from build123d import *

# Parameters (mm, degrees)
F0_R     = 11.2522
F1_DEPTH = 8.636


with BuildPart() as f1:
    # F0 (on Top) → F1 (new body)
    with BuildSketch(Plane.XY):
        with BuildLine():
            ThreePointArc((10.0592163849, -12.5427541219), (14.4955615296, -6.9560916599), (16.0782, 0))
            ThreePointArc((16.0782, 0), (15.9356487874, 2.1362614454), (15.5105229014, 4.2346422002))
            ThreePointArc((15.5105229014, 4.2346422002), (15.2912768803, 4.968437039), (15.0373368529, 5.6909591117))
            ThreePointArc((15.0373368529, 5.6909591117), (9.4505288434, 13.007537039), (0.7656311095, 16.0599602815))
            ThreePointArc((0.7656311095, 16.0599602815), (0, 16.0782), (-0.7656311095, 16.0599602815))
            ThreePointArc((-0.7656311095, 16.0599602815), (-9.4505288434, 13.007537039), (-15.0373368529, 5.6909591117))
            ThreePointArc((-15.0373368529, 5.6909591117), (-15.2912768803, 4.968437039), (-15.5105229014, 4.2346422002))
            ThreePointArc((-15.5105229014, 4.2346422002), (-15.2912768803, -4.968437039), (-10.0592163849, -12.5427541219))
            ThreePointArc((-10.0592163849, -12.5427541219), (-9.4505288434, -13.007537039), (-8.8203992269, -13.4428074716))
            ThreePointArc((-8.8203992269, -13.4428074716), (0, -16.0782), (8.8203992269, -13.4428074716))
            ThreePointArc((8.8203992269, -13.4428074716), (9.4505288434, -13.007537039), (10.0592163849, -12.5427541219))
        make_face()
        Circle(F0_R, mode=Mode.SUBTRACT)
        with BuildLine():
            ThreePointArc((0.7656311095, 16.0599602815), (9.4505288434, 13.007537039), (15.0373368529, 5.6909591117))
            ThreePointArc((15.0373368529, 5.6909591117), (15.1741938942, 5.3328401038), (15.3133632508, 4.9756133358))
            ThreePointArc((15.3133632508, 4.9756133358), (13.983030327, 11.6776288921), (13.4324519852, 18.4881840601))
            ThreePointArc((13.4324519852, 18.4881840601), (6.7850910488, 16.9072378917), (0, 16.1014229843))
            ThreePointArc((0, 16.1014229843), (0.3827485418, 16.079454203), (0.7656311095, 16.0599602815))
        make_face()
        with BuildLine():
            ThreePointArc((15.5105229014, 4.2346422002), (15.9356487874, 2.1362614454), (16.0782, 0))
            ThreePointArc((16.0782, 0), (14.4955615296, -6.9560916599), (10.0592163849, -12.5427541219))
            ThreePointArc((10.0592163849, -12.5427541219), (9.7609161203, -12.7835777623), (9.4641789711, -13.0263248279))
            ThreePointArc((9.4641789711, -13.0263248279), (15.4270790567, -9.6900663284), (21.7341638644, -7.0618579207))
            ThreePointArc((21.7341638644, -7.0618579207), (18.176447212, -1.2283812192), (15.3133632508, 4.9756133358))
            ThreePointArc((15.3133632508, 4.9756133358), (15.4107455022, 4.6048091142), (15.5105229014, 4.2346422002))
        make_face()
        with BuildLine():
            ThreePointArc((13.4324519852, 18.4881840601), (13.983030327, 11.6776288921), (15.3133632508, 4.9756133358))
            ThreePointArc((15.3133632508, 4.9756133358), (18.176447212, -1.2283812192), (21.7341638644, -7.0618579207))
            ThreePointArc((21.7341638644, -7.0618579207), (30.0130318433, -4.8169203604), (38.5291644649, -3.789844495))
            ThreePointArc((38.5291644649, -3.789844495), (22.4722564751, 7.3016787476), (28.9431341285, 25.7129232581))
            ThreePointArc((28.9431341285, 25.7129232581), (21.4497380646, 21.5381879262), (13.4324519852, 18.4881840601))
        make_face()
        with BuildLine():
            ThreePointArc((53.8417333554, 12.2701157865), (45.4020008846, 26.4179894446), (28.9431341285, 25.7129232581))
            ThreePointArc((28.9431341285, 25.7129232581), (22.4722564751, 7.3016787476), (38.5291644649, -3.789844495))
            ThreePointArc((38.5291644649, -3.789844495), (49.4000810682, 1.1751046298), (53.8417333554, 12.2701157865))
        make_face()
        with Locations((37.7635333554, 12.2701157865)):
            Circle(F0_R, mode=Mode.SUBTRACT)
        with BuildLine():
            ThreePointArc((21.7341638644, -7.0618579207), (15.4270790567, -9.6900663284), (9.4641789711, -13.0263248279))
            ThreePointArc((9.4641789711, -13.0263248279), (4.4485711229, -17.6664192363), (0, -22.8526522788))
            ThreePointArc((0, -22.8526522788), (4.693373395, -30.0325997603), (8.301810296, -37.8145392867))
            ThreePointArc((8.301810296, -37.8145392867), (13.8886183055, -19.1160431361), (33.3983635338, -19.5808260531))
            ThreePointArc((33.3983635338, -19.5808260531), (27.1123675633, -13.7442470619), (21.7341638644, -7.0618579207))
        make_face()
        with BuildLine():
            ThreePointArc((9.4641789711, -13.0263248279), (9.1416159705, -13.2335256587), (8.8203992269, -13.4428074716))
            ThreePointArc((8.8203992269, -13.4428074716), (0, -16.0782), (-8.8203992269, -13.4428074716))
            ThreePointArc((-8.8203992269, -13.4428074716), (-9.1416159705, -13.2335256587), (-9.4641789711, -13.0263248279))
            ThreePointArc((-9.4641789711, -13.0263248279), (-4.4485711229, -17.6664192363), (0, -22.8526522788))
            ThreePointArc((0, -22.8526522788), (4.4485711229, -17.6664192363), (9.4641789711, -13.0263248279))
        make_face()
        with BuildLine():
            ThreePointArc((-8.301810296, -37.8145392867), (-4.693373395, -30.0325997603), (0, -22.8526522788))
            ThreePointArc((0, -22.8526522788), (-4.4485711229, -17.6664192363), (-9.4641789711, -13.0263248279))
            ThreePointArc((-9.4641789711, -13.0263248279), (-15.4270790567, -9.6900663284), (-21.7341638644, -7.0618579207))
            ThreePointArc((-21.7341638644, -7.0618579207), (-27.1123675633, -13.7442470619), (-33.3983635338, -19.5808260531))
            ThreePointArc((-33.3983635338, -19.5808260531), (-16.3830554891, -17.6280186454), (-7.2609471489, -32.123580175))
            ThreePointArc((-7.2609471489, -32.123580175), (-7.5233034372, -35.0162610986), (-8.301810296, -37.8145392867))
        make_face()
        with BuildLine():
            ThreePointArc((-33.3983635338, -19.5808260531), (-32.7896759923, -45.131117214), (-8.301810296, -37.8145392867))
            ThreePointArc((-8.301810296, -37.8145392867), (-7.5233034372, -35.0162610986), (-7.2609471489, -32.123580175))
            ThreePointArc((-7.2609471489, -32.123580175), (-16.3830554891, -17.6280186454), (-33.3983635338, -19.5808260531))
        make_face()
        with Locations((-23.3391471489, -32.123580175)):
            Circle(F0_R, mode=Mode.SUBTRACT)
        with BuildLine():
            ThreePointArc((-9.4641789711, -13.0263248279), (-9.7609161203, -12.7835777623), (-10.0592163849, -12.5427541219))
            ThreePointArc((-10.0592163849, -12.5427541219), (-15.2912768803, -4.968437039), (-15.5105229014, 4.2346422002))
            ThreePointArc((-15.5105229014, 4.2346422002), (-15.4107455022, 4.6048091142), (-15.3133632508, 4.9756133358))
            ThreePointArc((-15.3133632508, 4.9756133358), (-18.176447212, -1.2283812192), (-21.7341638644, -7.0618579207))
            ThreePointArc((-21.7341638644, -7.0618579207), (-15.4270790567, -9.6900663284), (-9.4641789711, -13.0263248279))
        make_face()
        with BuildLine():
            ThreePointArc((39.4173471489, -32.123580175), (37.8347086786, -25.1674885151), (33.3983635338, -19.5808260531))
            ThreePointArc((33.3983635338, -19.5808260531), (13.8886183055, -19.1160431361), (8.301810296, -37.8145392867))
            ThreePointArc((8.301810296, -37.8145392867), (26.2318280725, -47.9394238868), (39.4173471489, -32.123580175))
        make_face()
        with Locations((23.3391471489, -32.123580175)):
            Circle(F0_R, mode=Mode.SUBTRACT)
        with BuildLine():
            ThreePointArc((-21.6853333554, 12.2701157865), (-23.6156596973, 19.9085833157), (-28.9431341285, 25.7129232581))
            ThreePointArc((-28.9431341285, 25.7129232581), (-53.0548102357, 17.2385528255), (-38.5291644649, -3.789844495))
            ThreePointArc((-38.5291644649, -3.789844495), (-26.6685221987, 0.6335680737), (-21.6853333554, 12.2701157865))
        make_face()
        with Locations((-37.7635333554, 12.2701157865)):
            Circle(F0_R, mode=Mode.SUBTRACT)
        with BuildLine():
            ThreePointArc((-15.3133632508, 4.9756133358), (-13.983030327, 11.6776288921), (-13.4324519852, 18.4881840601))
            ThreePointArc((-13.4324519852, 18.4881840601), (-21.4497380646, 21.5381879262), (-28.9431341285, 25.7129232581))
            ThreePointArc((-28.9431341285, 25.7129232581), (-23.6156596973, 19.9085833157), (-21.6853333554, 12.2701157865))
            ThreePointArc((-21.6853333554, 12.2701157865), (-26.6685221987, 0.6335680737), (-38.5291644649, -3.789844495))
            ThreePointArc((-38.5291644649, -3.789844495), (-30.0130318433, -4.8169203604), (-21.7341638644, -7.0618579207))
            ThreePointArc((-21.7341638644, -7.0618579207), (-18.176447212, -1.2283812192), (-15.3133632508, 4.9756133358))
        make_face()
        with BuildLine():
            ThreePointArc((-15.0373368529, 5.6909591117), (-9.4505288434, 13.007537039), (-0.7656311095, 16.0599602815))
            ThreePointArc((-0.7656311095, 16.0599602815), (-0.3827485418, 16.079454203), (0, 16.1014229843))
            ThreePointArc((0, 16.1014229843), (-6.7850910488, 16.9072378917), (-13.4324519852, 18.4881840601))
            ThreePointArc((-13.4324519852, 18.4881840601), (-13.983030327, 11.6776288921), (-15.3133632508, 4.9756133358))
            ThreePointArc((-15.3133632508, 4.9756133358), (-15.1741938942, 5.3328401038), (-15.0373368529, 5.6909591117))
        make_face()
        with BuildLine():
            ThreePointArc((0, 16.1014229843), (6.7850910488, 16.9072378917), (13.4324519852, 18.4881840601))
            ThreePointArc((13.4324519852, 18.4881840601), (13.8557003896, 27.0555792564), (15.5105229014, 35.4722865767))
            ThreePointArc((15.5105229014, 35.4722865767), (0, 23.628728777), (-15.5105229014, 35.4722865767))
            ThreePointArc((-15.5105229014, 35.4722865767), (-13.8557003896, 27.0555792564), (-13.4324519852, 18.4881840601))
            ThreePointArc((-13.4324519852, 18.4881840601), (-6.7850910488, 16.9072378917), (0, 16.1014229843))
        make_face()
        with BuildLine():
            ThreePointArc((-15.5105229014, 35.4722865767), (0, 23.628728777), (15.5105229014, 35.4722865767))
            ThreePointArc((15.5105229014, 35.4722865767), (15.9356487874, 37.5706673316), (16.0782, 39.706928777))
            ThreePointArc((16.0782, 39.706928777), (-2.1362614454, 55.6425775644), (-15.5105229014, 35.4722865767))
        make_face()
        with Locations((0, 39.706928777)):
            Circle(F0_R, mode=Mode.SUBTRACT)
    extrude(amount=F1_DEPTH)


solid = f1.part
Check sheet for the modelled part. Datum: model origin and axes. Units: mm. Coordinates: 2 decimals unless noted, no trailing zeros. Loops run counter-clockwise (first coordinate to the right, second up) from the corner with the lowest first, then second, coordinate; pieces in that order, holes last. Notation, with made-up numbers: (32.5, -2.75) -> (64.5, -2.75) arc R12 ccw to (64.5, 18.25) -> close; hole circle Ø8 at (18.5, 52). An arc over 180 degrees is marked (long way). Write item = value, one per line. Start each with the question number.
1. Draft check along Y on faces 1 (the cylindrical face through (-33.1, -44.9, 4.3)), 2 (the cylindrical face through (-21.341, 21.488, 4.258)), 3 (the flat face through (-13, 5, 0)). Enter one of: released by +Y, released by -Y, zero draft, split by the parting line, or undercut.
2. Section check C-C on z = 4. Give the number of separate pieces and of enclosed holes in the cut face, then the cut area to 3 significant figures.
3. Material ranges on line 1 (X direction, y = 11.5, z = 7); line 2 (X direction, y = -28, z = 6); line 3 (Y direction, x = -6.5, z = 2.5), recorded low to high.
4. Depth check by flat-ended pin: P1, Ø5, axis at x = -31, z = 2, coming from the -Y side; P2, Ø1.5, axis at x = 20.5, y = 10, coming from the -Z side; P3, Ø4, axis at x = 9.5, z = 8, coming from the +Y side. Enter the tip coordinate at first touch or a pass-through.
5. Section check A-A on y = -35.5. Record the cut outline in (x, z).
6. Section check B-B on x = 45. Record the cut outline in (y, z).
Responses:
q1.face_1 = undercut
q1.face_2 = undercut
q1.face_3 = zero draft
q2.separate_pieces = 1
q2.enclosed_holes = 11
q2.area = 3,950 mm2
q3.line_1 = -53.82 to -48.99, -26.54 to 26.54, 48.99 to 53.82
q3.line_2 = -38.88 to -33.81, -12.87 to -3.51, 3.51 to 12.87, 33.81 to 38.88
q3.line_3 = -33.56 to -9.18, 9.18 to 30.52, 48.89 to 54.41
q4.P1 = -47.35
q4.P2 = 0
q4.P3 = 53.93
q5.outline = (-39.06, 0) -> (-34.07, 0) -> (-34.07, 8.64) -> (-39.06, 8.64) -> close; (-12.61, 0) -> (-7.37, 0) -> (-7.37, 8.64) -> (-12.61, 8.64) -> close; (7.37, 0) -> (12.61, 0) -> (12.61, 8.64) -> (7.37, 8.64) -> close; (34.07, 0) -> (39.06, 0) -> (39.06, 8.64) -> (34.07, 8.64) -> close
q6.outline = (-2.09, 0) -> (3.65, 0) -> (3.65, 8.64) -> (-2.09, 8.64) -> close; (20.89, 0) -> (26.63, 0) -> (26.63, 8.64) -> (20.89, 8.64) -> close
